For this review, use the dimensioned drawing (mm, ordinates from the lowest corner) and the shaded views. Give positions to 0.01 mm unless a question says otherwise; leave off trailing zeros. Loops run counter-clockwise (first coordinate to the right, second up) from the corner with the lowest first, then second, coordinate; pieces in that order, holes last. Notation, with made-up numbers: (-2.75, 54) - (46.25, 54) arc R34 cw to (46.25, 86) - close; hole circle Ø10 at (37.25, 19.25). An arc over 180 degrees is marked (long way). Write each question's results on one line, items separated by ' | '.
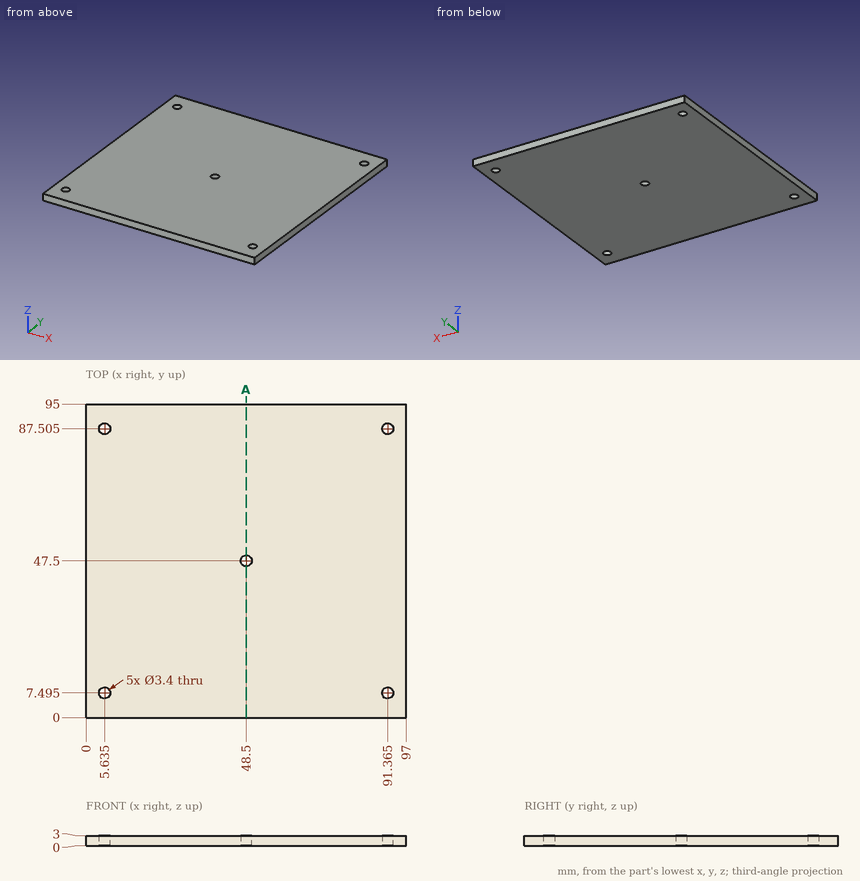
Item 1: Wall thickness on probe 1 along X at (y, z) = (8.5, 1.4); probe 2 along Y at (x, z) = (48.5, 1.2); probe 3 along X at (y, z) = (47.5, 1.6): over which ranges is each line inside the solid? List them lowest first.
Output values:
probe 1: x = 0 to 4.26, 7.01 to 89.99, 92.74 to 97 | probe 2: y = 0 to 45.8, 49.2 to 95 | probe 3: x = 0 to 46.8, 50.2 to 97
Item 2: We need section A-A on x = 48.5. Give the boundary of the cut face in (y, z), then the cut area to 3 significant figures.
Output values:
outline: (0, 0) - (45.8, 0) - (45.8, 3) - (0, 3) - close; (49.2, 0) - (95, 0) - (95, 3) - (49.2, 3) - close | area: 275 mm²
Item 3: Clearance check with a flat-ended pin moving along its axis: P1, Ø2, axis at x = 5.635, y = 7.495, coming from the -Z side. State where the tip first meets the part, or that it passes through.
Output values:
P1: passes through
